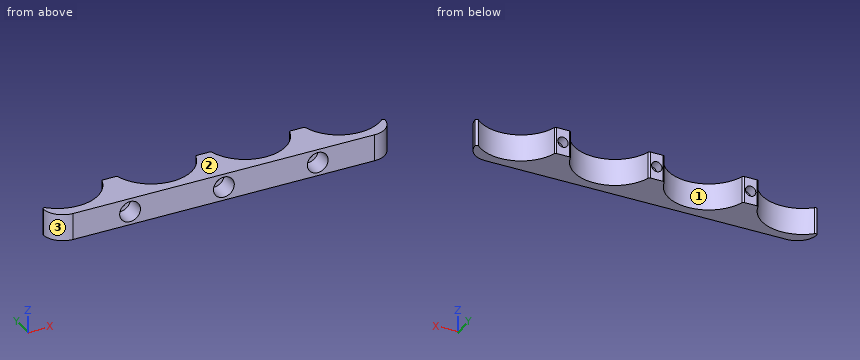
```python
from build123d import *

# Parameters (mm, degrees)
BOSS_EXTRU_1_DEPTH         = 4
CONG_1_R                   = 6
CONG_2_R                   = 0.5
R_P_TITION_LIN_AIRE1_COUNT = 3
R_P_TITION_LIN_AIRE1_PITCH = 28


with BuildPart() as part:
    # Esquisse1 → Boss.-Extru.1 (new, symmetric)
    with BuildSketch(Plane.XY):
        with BuildLine():
            Line((-30.277798842, 12), (-25.722201158, 12))
            ThreePointArc((-25.722201158, 12), (-14, 2.9), (-2.277798842, 12))
            Line((-2.277798842, 12), (2.277798842, 12))
            ThreePointArc((2.277798842, 12), (14, 2.9), (25.722201158, 12))
            Line((25.722201158, 12), (30.277798842, 12))
            ThreePointArc((30.277798842, 12), (39.114930254, 3.24898419), (51, 6.912355102))
            Line((51, 6.912355102), (51, 0))
            Line((51, 0), (-51, 0))
            Line((-51, 0), (-51, 6.912355102))
            ThreePointArc((-51, 6.912355102), (-39.114930254, 3.24898419), (-30.277798842, 12))
        make_face()
    extrude(amount=BOSS_EXTRU_1_DEPTH, both=True)

    # Congé1
    cong_1_edges = [part.edges().sort_by_distance(p)[0] for p in [
        (51, 0, 0),
        (-51, 0, 0),
    ]]
    fillet(cong_1_edges, radius=CONG_1_R)

    # Congé2
    cong_2_edges = [part.edges().sort_by_distance(p)[0] for p in [
        (51, 6.912355102, 0),
        (30.277798842, 12, 0),
        (25.722201158, 12, 0),
        (2.277798842, 12, 0),
        (-2.277798842, 12, 0),
        (-25.722201158, 12, 0),
        (-30.277798842, 12, 0),
        (-51, 6.912355102, 0),
    ]]
    fillet(cong_2_edges, radius=CONG_2_R)

    # Esquisse2 → Enlèvement de matière-Révolution1 (revolve, cut)
    with BuildSketch(Plane.XY, mode=Mode.PRIVATE) as enl_vement_de_mati_re_r_volution1_sk:
        Polygon((-28, 12), (-28, 0), (-24.9, 0), (-24.9, 5.8), (-26.1, 5.8), (-26.1, 9), (-26.45, 9), (-26.45, 12), align=None)
    enl_vement_de_mati_re_r_volution1 = revolve(enl_vement_de_mati_re_r_volution1_sk.sketch.rotate(Axis((-28, 0, 0), (0, -1, 0)), 90), axis=Axis((-28, 0, 0), (0, -1, 0)), mode=Mode.SUBTRACT)

    # Répétition linéaire1: Enlèvement de matière-Révolution1 ×3
    with Locations(*[(i * R_P_TITION_LIN_AIRE1_PITCH, 0, 0) for i in range(1, R_P_TITION_LIN_AIRE1_COUNT)]):
        add(enl_vement_de_mati_re_r_volution1, mode=Mode.SUBTRACT)


solid = part.part
```
Verification items for the finished model (mm, model axes). Face numbers are marked on the shaded views. Round coordinates to 2 decimals unless told otherwise and drop trailing zeros. Write each loop counter-clockwise with the first axis right and the second up, starting at its lowest first coordinate (ties: lowest second). Pieces come first, ordered by that corner, then holes. Notation, with made-up numbers: (48, 88.5) - (82, 88.5) arc R18 ccw to (82, 122.5) - close; hole circle Ø5 at (34, -17.5). An arc over 180 degrees is marked (long way). Answer as a JSON object with one key per item and string values. Group by question number.
Q1. Section check C-C, the plane y = 4. Enter the section's corners in (x, z), plus the area to 3 significant figures.
Q2. Go/stop test with flat-tipped pins: pin 1 Ø3 at (x, z) = (-28, 0) entering from +Y; pin 2 Ø1.5 at (y, z) = (7.5, 0.5) entering from -X; pin 3 Ø4 at (x, z) = (-27.5, -0.5) entering from -Y; pin 4 Ø2 at (y, z) = (7, -2) entering from -X. Record where each tip stops, or that it passes through.
Q3. Section check D-D, the plane z = 0. Give the number of separate pieces and of enclosed holes in the cut face, plus the area to 3 significant figures.
Q4. Thickness scan on line 1 (Z direction, x = 28, y = 2.7); line 2 (X direction, y = 7.75, z = 3.5); line 3 (Z direction, x = 28, y = 7.9). Record the ranges inside material, lowest first.
Q5. Mould release check, pull along X, two halves, no side actions. Record for the marked faces 1, 2 and 3: released by +X, released by -X, zero draft, split by the parting line, or undercut.
Q6. Section check B-B, the plane x = 28. Enter the section's corners in (y, z), plus the area to 3 significant figures.
Q7. Section check A-A, the plane y = 7.75. Enter the section's corners in (x, z), plus the area to 3 significant figures.
Found:
{
 "1": {"outline": "(-50.66, -4) - (-47.04, -4) - (-47.04, 4) - (-50.66, 4) - close; (-36.96, -4) - (-19.04, -4) - (-19.04, 4) - (-36.96, 4) - close; (-8.96, -4) - (8.96, -4) - (8.96, 4) - (-8.96, 4) - close; (19.04, -4) - (36.96, -4) - (36.96, 4) - (19.04, 4) - close; (47.04, -4) - (50.66, -4) - (50.66, 4) - (47.04, 4) - close; hole circle Ø6.2 at (-28, 0); hole circle Ø6.2 at (0, 0); hole circle Ø6.2 at (28, 0)", "area": "397 mm^2"},
 "2": {"pin 1": "passes through", "pin 2": "stops at x = -33.15", "pin 3": "stops at y = 5.8", "pin 4": "stops at x = -50.88"},
 "3": {"separate pieces": "4", "enclosed holes": "0", "area": "420 mm^2"},
 "4": {"line 1": "z = -4 to -3.1, 3.1 to 4", "line 2": "x = -32.31 to -23.69, -4.31 to 4.31, 23.69 to 32.31", "line 3": "z = -4 to -1.9, 1.9 to 4"},
 "5": {"face 1": "undercut", "face 2": "zero draft", "face 3": "released by -X"},
 "6": {"outline": "(0, -4) - (12, -4) - (12, -1.55) - (9, -1.55) - (9, -1.9) - (5.8, -1.9) - (5.8, -3.1) - (0, -3.1) - close; (0, 3.1) - (5.8, 3.1) - (5.8, 1.9) - (9, 1.9) - (9, 1.55) - (12, 1.55) - (12, 4) - (0, 4) - close", "area": "38.6 mm^2"},
 "7": {"outline": "(-32.31, -4) - (-23.69, -4) - (-23.69, 4) - (-32.31, 4) - close; (-4.31, -4) - (4.31, -4) - (4.31, 4) - (-4.31, 4) - close; (23.69, -4) - (32.31, -4) - (32.31, 4) - (23.69, 4) - close; hole circle Ø3.8 at (-28, 0); hole circle Ø3.8 at (0, 0); hole circle Ø3.8 at (28, 0)", "area": "173 mm^2"}
}
